```python
from build123d import *

# Parameters (mm, degrees)
SKETCH_1_R      = 11.05
SKETCH_1_R_2    = 2.75
SKETCH_1_R_3    = 1.25
SKETCH_1_R_4    = 4.25
EXTRUDE_1_DEPTH = 3


with BuildPart() as part:
    # 草图1 → 凸台-拉伸1 (new body)
    with BuildSketch(Plane.XY):
        with BuildLine():
            Line((-40, 20), (-40, -37))
            ThreePointArc((-40, -37), (-38.535533906, -40.535533906), (-35, -42))
            Line((-35, -42), (35, -42))
            ThreePointArc((35, -42), (38.535533906, -40.535533906), (40, -37))
            Line((40, -37), (40, 20))
            ThreePointArc((40, 20), (38.535533906, 23.535533906), (35, 25))
            Line((35, 25), (-35, 25))
            ThreePointArc((-35, 25), (-38.535533906, 23.535533906), (-40, 20))
        make_face()
        Circle(SKETCH_1_R, mode=Mode.SUBTRACT)
        with Locations((-25, 16)):
            Circle(SKETCH_1_R_2, mode=Mode.SUBTRACT)
        with Locations((-25, -16)):
            Circle(SKETCH_1_R_2, mode=Mode.SUBTRACT)
        with Locations((25, -16)):
            Circle(SKETCH_1_R_2, mode=Mode.SUBTRACT)
        with Locations((25, 16)):
            Circle(SKETCH_1_R_2, mode=Mode.SUBTRACT)
        with Locations((0, -32)):
            Circle(SKETCH_1_R_3, mode=Mode.SUBTRACT)
        with Locations((-20, -32)):
            Circle(SKETCH_1_R_3, mode=Mode.SUBTRACT)
        with Locations((20, -32)):
            Circle(SKETCH_1_R_3, mode=Mode.SUBTRACT)
        with Locations((-25, 0)):
            Circle(SKETCH_1_R_4, mode=Mode.SUBTRACT)
        with Locations((25, 0)):
            Circle(SKETCH_1_R_4, mode=Mode.SUBTRACT)
        with Locations((-14.1, 15.5)):
            Circle(SKETCH_1_R_3, mode=Mode.SUBTRACT)
        with Locations((14.1, 15.5)):
            Circle(SKETCH_1_R_3, mode=Mode.SUBTRACT)
        with Locations((14.1, -15.5)):
            Circle(SKETCH_1_R_3, mode=Mode.SUBTRACT)
        with Locations((-14.1, -15.5)):
            Circle(SKETCH_1_R_3, mode=Mode.SUBTRACT)
    extrude(amount=EXTRUDE_1_DEPTH)


solid = part.part
```
Geometry: final body of the model. Coordinates: model frame, mm. Round coordinates to 2 decimals unless told otherwise and drop trailing zeros. Loops run counter-clockwise (first coordinate to the right, second up) from the corner with the lowest first, then second, coordinate; pieces in that order, holes last.
Item 1: Section D-D, the plane x = -24. Output: boundary loops of the cut face in (y, z), plus the area to 3 significant figures.
Checked values:
outline: (-42, 0) - (-18.56, 0) - (-18.56, 3) - (-42, 3) - close; (-13.44, 0) - (-4.13, 0) - (-4.13, 3) - (-13.44, 3) - close; (4.13, 0) - (13.44, 0) - (13.44, 3) - (4.13, 3) - close; (18.56, 0) - (25, 0) - (25, 3) - (18.56, 3) - close
area: 145 mm2
Item 2: Contact query for a flat-ended pin moving along its axis: P1, Ø4.5, axis at x = -25, y = -16, coming from the +Z side (3 decimals). Output: stop coordinate, or through.
Checked values:
P1: passes through
Item 3: Mould query, pull axis Y, two halves, no side actions, for faces 1 (the cylindrical face through (-38, 24, 1)), 2 (the cylindrical face through (21.868, 2.872, 1.479)), 3 (the flat face through (-40, -8, 1)). Classes: released by +Y, released by -Y, zero draft, split by the parting line, or undercut.
Checked values:
face 1: released by +Y
face 2: undercut
face 3: zero draft
Item 4: Line query: L1, parallel to Y at x = -14.1, z = 2.1; L2, parallel to Y at x = 0, z = 1.45; L3, parallel to Y at x = 25, z = 1.2. Output: solid intervals per line, ascending.
Checked values:
L1: y = -42 to -16.75, -14.25 to 14.25, 16.75 to 25
L2: y = -42 to -33.25, -30.75 to -11.05, 11.05 to 25
L3: y = -42 to -18.75, -13.25 to -4.25, 4.25 to 13.25, 18.75 to 25
Item 5: Section C-C, the plane z = 0.45. State how many separate pieces and enclosed holes the cut face has, plus the area to 3 significant figures.
Checked values:
separate pieces: 1
enclosed holes: 14
area: 4,710 mm2
Item 6: Section A-A, the plane x = 14.1. Output: boundary loops of the cut face in (y, z).
Checked values:
outline: (-42, 0) - (-16.75, 0) - (-16.75, 3) - (-42, 3) - close; (-14.25, 0) - (14.25, 0) - (14.25, 3) - (-14.25, 3) - close; (16.75, 0) - (25, 0) - (25, 3) - (16.75, 3) - close
Item 7: Section B-B, the plane y = -32. Output: boundary loops of the cut face in (x, z).
Checked values:
outline: (-40, 0) - (-21.25, 0) - (-21.25, 3) - (-40, 3) - close; (-18.75, 0) - (-1.25, 0) - (-1.25, 3) - (-18.75, 3) - close; (1.25, 0) - (18.75, 0) - (18.75, 3) - (1.25, 3) - close; (21.25, 0) - (40, 0) - (40, 3) - (21.25, 3) - close
